Autodesk Inventor part; units mm, degrees
ref_plane "YZ Plane" through (0, 0, 0) normal (1, 0, 0) x (0, 1, 0)
ref_plane "XZ Plane" through (0, 0, 0) normal (0, 1, 0) x (-1, 0, 0)
ref_plane "XY Plane" through (0, 0, 0) normal (0, 0, 1) x (1, 0, 0)
sketch "Sketch2" plane through (0, 0, 0) normal (1, 0, 0) x (0, 1, 0)
  line L0 (0, -26.67) -> (0, 26.67) construction
  line L1 (-26.67, 0) -> (26.67, 0) construction
  line L2 (17.4625, 17.4625) -> (-17.4625, 17.4625)
  line L3 (-17.4625, 17.4625) -> (-17.4625, -17.4625)
  line L4 (-17.4625, -17.4625) -> (17.4625, -17.4625)
  line L5 (17.4625, -17.4625) -> (17.4625, 17.4625)
  line L6 (19.05, 19.05) -> (-19.05, 19.05)
  line L7 (-19.05, 19.05) -> (-19.05, -19.05)
  line L8 (-19.05, -19.05) -> (19.05, -19.05)
  line L9 (19.05, -19.05) -> (19.05, 19.05)
  point P0 (0, 0)
  point P1 (0, 19.05)
  point P2 (0, 17.4625)
  point P3 (17.4625, 0)
  point P4 (19.05, 0)
  dimension "d0" = 1.5875
  dimension "d1" = 38.1
extrude "Extrusion1" add sketch "Sketch2" along normal mid plane 457.2
sketch "Sketch3" plane through (-228.6, -19.05, 19.05) normal (0, 0, 1) x (1, 0, 0)
  line L0 (-91.44, 19.05) -> (548.64, 19.05) construction
  line L1 (228.6, -7.62) -> (228.6, 45.72) construction
  circle A0 centre (12.7, 19.05) radius 7.9375
  line L2 (0, 0) -> (0, 38.1) construction
  circle A1 centre (444.5, 19.05) radius 7.9375
  point P0 (228.6, 19.05)
  dimension "d4" = 12.7
  dimension "d5" = 15.875
extrude "Extrusion2" cut sketch "Sketch3" against normal through all
sketch "Sketch5" plane through (-228.6, 19.05, 19.05) normal (0, 1, 0) x (1, 0, 0)
  circle A0 centre (228.6, 19.05) radius 14.2875
  dimension "d11" = 28.575
extrude "Extrusion4" cut sketch "Sketch5" against normal through all
sketch "Sketch6" plane through (-228.6, 19.05, 19.05) normal (0, 1, 0) x (1, 0, 0)
  line L0 (-91.44, 19.05) -> (548.64, 19.05) construction
  line L1 (228.6, 45.72) -> (228.6, -7.62) construction
  circle A0 centre (209.55, 19.05) radius 3.175 construction
  circle A1 centre (247.65, 19.05) radius 3.175 construction
  circle A2 centre (228.6, 19.05) radius 15.875 construction
  circle A3 centre (209.55, 19.05) radius 2.667
  circle A4 centre (247.65, 19.05) radius 2.667
  dimension "d14" = 31.75
  dimension "d15" = 6.35
  dimension "d16" = 5.334
extrude "Extrusion5" cut sketch "Sketch6" against normal through all
properties part number "Crossbeam" material "Aluminum 6061"
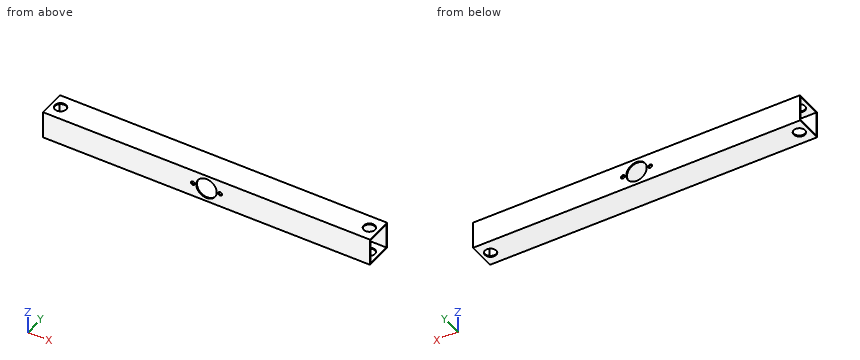
Can you work these out from the model? Positions are in its coordinate system, mm. Coordinates: 2 decimals unless noted, no trailing zeros. Loops run counter-clockwise (first coordinate to the right, second up) from the corner with the lowest first, then second, coordinate; pieces in that order, holes last. Notation, with made-up numbers: (32, -40) - (67, -40) arc R18 cw to (67, -8) - close; hole circle Ø9 at (6.25, 70.5). An arc over 180 degrees is marked (long way). Put each result on its own line as item: value. Start each with the question number.
Item 1: Suppose I cut it at C-C (x = 215.9). Please give me the cut outline in (y, z), and give its area (3 significant figures).
Item 2: Suppose I cut it at B-B (y = 0). Please give me the cut outline in (x, z).
Item 3: Suppose I cut it at A-A (x = 0). Please give me the cut outline in (y, z).
Item 4: If I drill on line 1 along X through (y, z) = (-18.3, 0); line 2 along Y through (x, z) = (-57.5, -10.5), over which ranges is the centre line in solid material (lowest first)?
Item 5: For pin 1 (8.5 mm diameter, centred on x = 19.05, z = 0, fed in from -Y), with a flat end and sliding along its axis, tell me the tip position at first contact or that it passes through.
Here are the results:
1. outline: (-19.05, -19.05) - (-7.94, -19.05) - (-7.94, -17.46) - (-17.46, -17.46) - (-17.46, 17.46) - (-7.94, 17.46) - (-7.94, 19.05) - (-19.05, 19.05) - close; (7.94, -19.05) - (19.05, -19.05) - (19.05, 19.05) - (7.94, 19.05) - (7.94, 17.46) - (17.46, 17.46) - (17.46, -17.46) - (7.94, -17.46) - close
1. area: 181 mm²
2. outline: (-228.6, -19.05) - (-223.84, -19.05) - (-223.84, -17.46) - (-228.6, -17.46) - close; (-228.6, 17.46) - (-223.84, 17.46) - (-223.84, 19.05) - (-228.6, 19.05) - close; (-207.96, -19.05) - (207.96, -19.05) - (207.96, -17.46) - (-207.96, -17.46) - close; (-207.96, 17.46) - (207.96, 17.46) - (207.96, 19.05) - (-207.96, 19.05) - close; (223.84, -19.05) - (228.6, -19.05) - (228.6, -17.46) - (223.84, -17.46) - close; (223.84, 17.46) - (228.6, 17.46) - (228.6, 19.05) - (223.84, 19.05) - close
3. outline: (-19.05, -19.05) - (19.05, -19.05) - (19.05, -14.29) - (17.46, -14.29) - (17.46, -17.46) - (-17.46, -17.46) - (-17.46, -14.29) - (-19.05, -14.29) - close; (-19.05, 14.29) - (-17.46, 14.29) - (-17.46, 17.46) - (17.46, 17.46) - (17.46, 14.29) - (19.05, 14.29) - (19.05, 19.05) - (-19.05, 19.05) - close
4. line 1: -228.6 to -21.72, -16.38 to -14.29, 14.29 to 16.38, 21.72 to 228.6
4. line 2: -19.05 to -17.46, 17.46 to 19.05
5. pin 1: y = -19.05
